Read the model definition and answer for the solid it produces. Units are mm, in the model's axes. A direction names the side the tool comes from. Round coordinates to 2 decimals unless told otherwise and drop trailing zeros. Loops run counter-clockwise (first coordinate to the right, second up) from the corner with the lowest first, then second, coordinate; pieces in that order, holes last. Notation, with made-up numbers: M 67.25,62.25 L 84.25,62.25 A15 ccw 84.25,72.25 Z; hole C 2.25,20 d5. An arc over 180 degrees is marked long. Write each question's results on one line, items separated by ' | '.
from build123d import *

# Parameters (mm, degrees)
BOSS_EXTRUDE1_DEPTH = 5
BOSS_EXTRUDE2_DEPTH = 20
BOSS_EXTRUDE3_DEPTH = 50
SKETCH2_W           = 28.5
SKETCH2_H           = 1
BOSS_EXTRUDE4_DEPTH = 1.4
SKETCH2_3_W         = 1.5
SKETCH2_3_H         = 1
BOSS_EXTRUDE5_DEPTH = 15


with BuildPart() as part:
    # Sketch1 → Boss-Extrude1 (new body)
    with BuildSketch(Plane(origin=(0, 0, 0), x_dir=(1, 0, 0), z_dir=(0, 1, 0))):
        Polygon((0, 80), (-30, 80), (-30, 7), (-30, 0), (0, 0), align=None)
    extrude(amount=BOSS_EXTRUDE1_DEPTH)

    # Sketch1<3> → Boss-Extrude2 (add)
    with BuildSketch(Plane(origin=(0, 0, 0), x_dir=(1, 0, 0), z_dir=(0, 1, 0))):
        Polygon((-35, 85), (-35, 7), (-30, 7), (-30, 80), (0, 80), (0, 85), align=None)
    extrude(amount=BOSS_EXTRUDE2_DEPTH)

    # Sketch1<4> → Boss-Extrude3 (add)
    with BuildSketch(Plane(origin=(0, 0, 0), x_dir=(1, 0, 0), z_dir=(0, 1, 0))):
        Polygon((-30, 0), (-30, 7), (-35, 7), (-80, 7), (-80, 0), align=None)
    extrude(amount=BOSS_EXTRUDE3_DEPTH)

    # Sketch2 → Boss-Extrude4 (add)
    with BuildSketch(Plane(origin=(0, 5, 0), x_dir=(1, 0, 0), z_dir=(0, 1, 0))):
        with Locations((-14.25, 0.5)):
            Rectangle(SKETCH2_W, SKETCH2_H)
    extrude(amount=BOSS_EXTRUDE4_DEPTH)

    # Sketch2<3> → Boss-Extrude5 (add)
    with BuildSketch(Plane(origin=(0, 5, 0), x_dir=(1, 0, 0), z_dir=(0, 1, 0))):
        with Locations((-29.25, 0.5)):
            Rectangle(SKETCH2_3_W, SKETCH2_3_H)
    extrude(amount=BOSS_EXTRUDE5_DEPTH)


solid = part.part
Item 1: The part is cut by section A-A (x = -19). Determine the outline of the cut face in (y, z), plus the area to 3 significant figures.
Outcome:
outline: M 0,-85 L 20,-85 L 20,-80 L 5,-80 L 5,-1 L 6.4,-1 L 6.4,0 L 0,0 Z | area: 501 mm2
Item 2: The part is cut by section B-B (z = -36). Determine the outline of the cut face in (x, y), plus the area to 3 significant figures.
Outcome:
outline: M -35,0 L 0,0 L 0,5 L -30,5 L -30,20 L -35,20 Z | area: 250 mm2
Item 3: The part is cut by section D-D (x = -43.5). Determine the outline of the cut face in (y, z), plus the area to 3 significant figures.
Outcome:
outline: M 0,-7 L 50,-7 L 50,0 L 0,0 Z | area: 350 mm2
Item 4: Flat-ended cylindrical pins translate along their axes: pin 1 (8 mm diameter, centred on x = -59, y = 22, fed in from -Z); pin 2 (6 mm diameter, centred on y = 10.5, z = -58, fed in from -X); pin 3 (1.1 mm diameter, centred on y = 14, z = -0.5, fed in from +X). Find the tip coordinate at first contact, or state that the pin passes through.
Outcome:
pin 1: stops at z = -7 | pin 2: stops at x = -35 | pin 3: stops at x = -28.5
Item 5: Straight lines are drawn through the part: line 1 (Z direction, x = -22, y = 6); line 2 (Z direction, x = -60, y = 3); line 3 (Y direction, x = -10, z = -35). For each, find the intervals that lie inside material, in ascending order.
Outcome:
line 1: z = -85 to -80, -1 to 0 | line 2: z = -7 to 0 | line 3: y = 0 to 5
Item 6: The mould has two halves that part along Z. Classify faces 6 (the face through (-55, 50, -4)), 7 (the face through (-17, 10, -85)), 8 (the face through (-18, 6, -1)): pulls with the +Z half, pulls with the -Z half, needs draft (parallel to the pull), parting line crosses it, or undercut.
Outcome:
face 6: needs draft | face 7: pulls with the -Z half | face 8: undercut
Item 7: The part is cut by section C-C (y = 13.5). Determine the outline of the cut face in (x, z).
Outcome:
outline: M -80,-7 L -35,-7 L -35,-85 L 0,-85 L 0,-80 L -30,-80 L -30,-1 L -28.5,-1 L -28.5,0 L -80,0 Z
Item 8: For faces 1 (the face through (-31, 20, -55)), 2 (the face through (-35, 10, -47)), 3 (the face through (-80, 25, -4)), 4 (the face through (-49, 25, 0)), 5 (the face through (-15, 5, -41)), determine the directions among +Z, -Z, +X, -X, +Y, -Y from which every point of the face is accessible in a straight line to the end or side of a thin tool.
Outcome:
face 1: -Z, +X, -X, +Y | face 2: -Z, -X, +Y, -Y | face 3: +Z, -Z, -X, +Y, -Y | face 4: +Z, +X, -X, +Y, -Y | face 5: +X, +Y
